from build123d import *

# Parameters (mm, degrees)
SKETCH1_W           = 20
SKETCH1_H           = 20
SKETCH1_W_2         = 16
SKETCH1_H_2         = 16
BOSS_EXTRUDE1_DEPTH = 210
SKETCH2_R           = 2.5
CUT_EXTRUDE1_DEPTH  = 212.187120819
SKETCH3_R           = 2
CUT_EXTRUDE2_DEPTH  = 212.187120819


with BuildPart() as part:
    # Sketch1 → Boss-Extrude1 (new body)
    with BuildSketch(Plane.XY):
        Rectangle(SKETCH1_W, SKETCH1_H)
        Rectangle(SKETCH1_W_2, SKETCH1_H_2, mode=Mode.SUBTRACT)
    extrude(amount=BOSS_EXTRUDE1_DEPTH)

    # Sketch2 → Cut-Extrude1 (cut, through all)
    with BuildSketch(Plane(origin=(0, 10, 0), x_dir=(1, 0, 0), z_dir=(0, 1, 0))):
        with Locations(Location((0, -10, 0), (0, 0, 270))):
            Circle(SKETCH2_R)
        with Locations(Location((0, -30, 0), (0, 0, 270))):
            Circle(SKETCH2_R)
        with Locations(Location((0, -200, 0), (0, 0, 270))):
            Circle(SKETCH2_R)
        with Locations(Location((0, -180, 0), (0, 0, 270))):
            Circle(SKETCH2_R)
    extrude(amount=-CUT_EXTRUDE1_DEPTH, mode=Mode.SUBTRACT)

    # Sketch3 → Cut-Extrude2 (cut, through all)
    with BuildSketch(Plane(origin=(0, 10, 0), x_dir=(1, 0, 0), z_dir=(0, 1, 0))):
        with Locations(Location((-5, -70, 0), (0, 0, 270))):
            Circle(SKETCH3_R)
        with Locations(Location((5, -70, 0), (0, 0, 270))):
            Circle(SKETCH3_R)
        with Locations(Location((5, -140, 0), (0, 0, 270))):
            Circle(SKETCH3_R)
        with Locations(Location((-5, -140, 0), (0, 0, 270))):
            Circle(SKETCH3_R)
    extrude(amount=-CUT_EXTRUDE2_DEPTH, mode=Mode.SUBTRACT)


solid = part.part
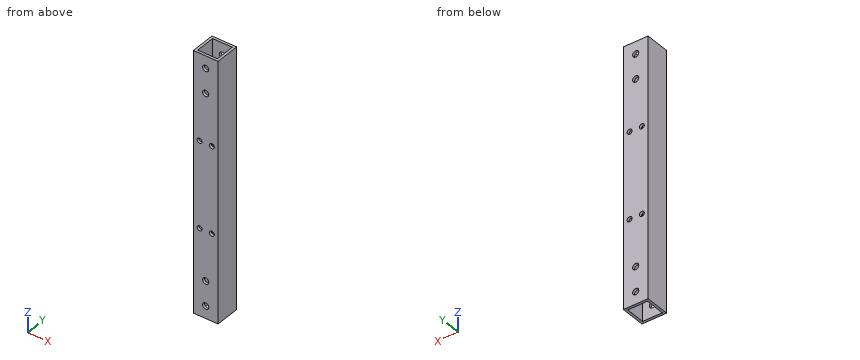
Design review of the part built by this model. Coordinates are the model's own, in mm. Round coordinates to 2 decimals unless told otherwise and drop trailing zeros. Loops run counter-clockwise (first coordinate to the right, second up) from the corner with the lowest first, then second, coordinate; pieces in that order, holes last. Notation, with made-up numbers: (-16.75, 69) - (-7.75, 69) arc R12 cw to (-7.75, 86) - close; hole circle Ø4 at (-13, -14). An arc over 180 degrees is marked (long way). One line per question, with ' | ' between items.
1. We need section A-A, the plane x = -5. State the section outline as (y, z) points, and give its area (3 significant figures).
Results are:
outline: (-10, 0) - (-8, 0) - (-8, 68) - (-10, 68) - close; (-10, 72) - (-8, 72) - (-8, 138) - (-10, 138) - close; (-10, 142) - (-8, 142) - (-8, 210) - (-10, 210) - close; (8, 0) - (10, 0) - (10, 68) - (8, 68) - close; (8, 72) - (10, 72) - (10, 138) - (8, 138) - close; (8, 142) - (10, 142) - (10, 210) - (8, 210) - close | area: 808 mm²
2. Clearance check with a flat-ended pin moving along its axis: P1, Ø2.5, axis at x = 5, z = 140, coming from the +Y side. State where the tip first meets the part, or that it passes through.
Results are:
P1: passes through
3. We need section D-D, the plane z = 180. State the section outline as (x, y) points.
Results are:
outline: (-10, -10) - (-2.5, -10) - (-2.5, -8) - (-8, -8) - (-8, 8) - (-2.5, 8) - (-2.5, 10) - (-10, 10) - close; (2.5, -10) - (10, -10) - (10, 10) - (2.5, 10) - (2.5, 8) - (8, 8) - (8, -8) - (2.5, -8) - close
4. We need section B-B, the plane z = 124.5. State the section outline as (x, y) points.
Results are:
outline: (-10, -10) - (10, -10) - (10, 10) - (-10, 10) - close; hole (-8, -8) - (8, -8) - (8, 8) - (-8, 8) - close
5. For L1, parallel to X at y = 8.4, z = 140; L2, parallel to X at y = -9.35, z = 180; L3, parallel to Y at x = -1, z = 79, list the stretches that pass through material, from the lowest coordinate up. Write a range as [from, to].
Results are:
L1: x = [-10, -7], [-3, 3], [7, 10] | L2: x = [-10, -2.5], [2.5, 10] | L3: y = [-10, -8], [8, 10]
6. We need section C-C, the plane y = -5.5. State the section outline as (x, z) points, and give its area (3 significant figures).
Results are:
outline: (-10, 0) - (-8, 0) - (-8, 210) - (-10, 210) - close; (8, 0) - (10, 0) - (10, 210) - (8, 210) - close | area: 840 mm²
